Geometry: see drawing. Coordinates: mm, zero at the bounding-box minimum. Give positions to 0.01 mm unless a question says otherwise; leave off trailing zeros. Order: outer loops, then holes, each group sorted by start corner. A loop starts at its lowest first (then second) coordinate and runs counter-clockwise, first axis right, second up. Notation, with made-up numbers: (79, 29.25) - (131, 29.25) arc R25 cw to (131, 47.25) - close; hole circle Ø10 at (57, 36). An arc over 180 degrees is marked (long way). One line per item, written item: value.
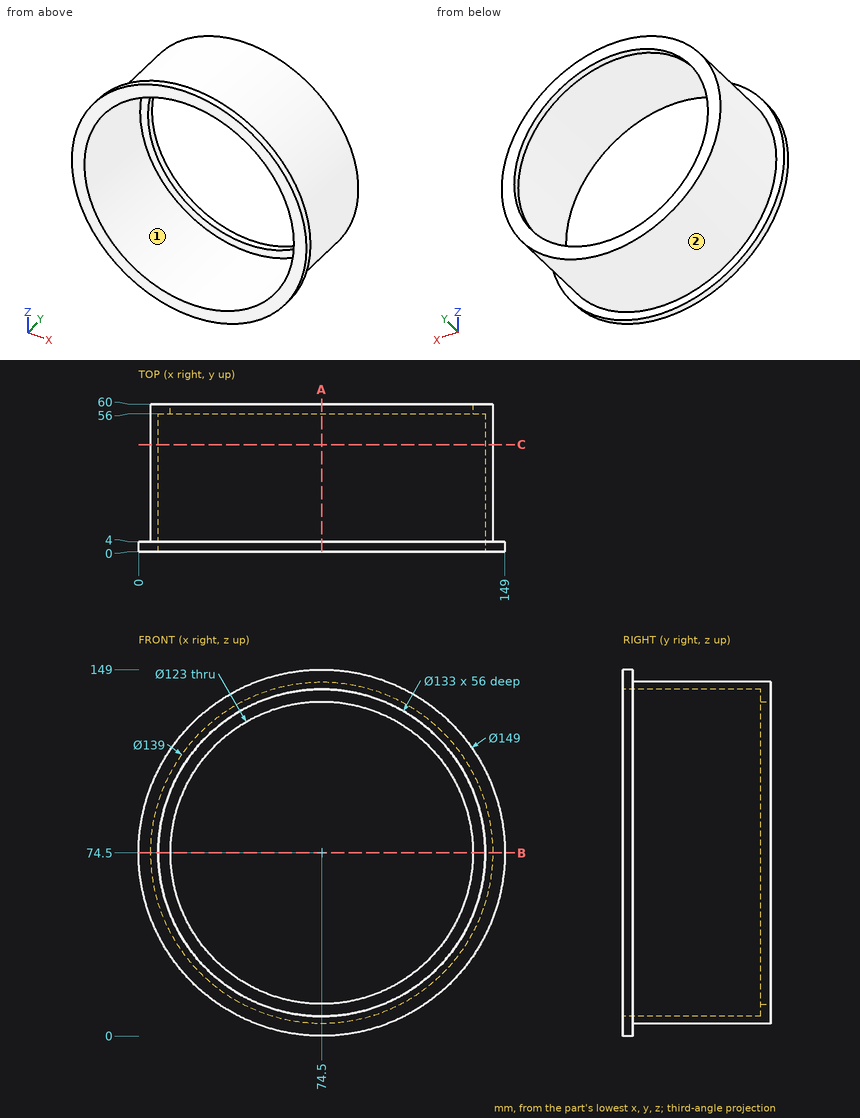
1) Section B-B, the plane z = 74.5. Return loops of the section in (x, y), then the cut area to 3 significant figures.
Answers below:
outline: (0, 0) - (8, 0) - (8, 56) - (13, 56) - (13, 60) - (5, 60) - (5, 4) - (0, 4) - close; (136, 56) - (141, 56) - (141, 0) - (149, 0) - (149, 4) - (144, 4) - (144, 60) - (136, 60) - close
area: 440 mm^2
2) First-contact query: pin 1 (1.5 mm diameter, centred on y = 16, z = 106.5, fed in from -X); pin 2 (1.5 mm diameter, centred on x = 100, y = 38.5, fed in from +Z); pin 3 (5 mm diameter, centred on y = 14, z = 48.5, fed in from -X). Flat tips, straight axial feed; report the tip coordinate or a pass-through.
Answers below:
pin 1: x = 12.42
pin 2: z = 139.44
pin 3: x = 9.09
3) Section A-A, the plane x = 74.5. Return loops of the section in (y, z), then the cut area to 3 significant figures.
Answers below:
outline: (0, 0) - (4, 0) - (4, 5) - (60, 5) - (60, 13) - (56, 13) - (56, 8) - (0, 8) - close; (0, 141) - (56, 141) - (56, 136) - (60, 136) - (60, 144) - (4, 144) - (4, 149) - (0, 149) - close
area: 440 mm^2
4) Material intervals for line 1 along Z through (x, y) = (74.5, 58.4); line 2 along Z through (x, y) = (74.5, 35.5), sorted ascending.
Answers below:
line 1: 5 to 13, 136 to 144
line 2: 5 to 8, 141 to 144
5) Section C-C, the plane y = 43.5. Return loops of the section in (x, z).
Answers below:
outline: circle Ø139 at (74.5, 74.5); hole circle Ø133 at (74.5, 74.5)
6) Mould query, pull axis Z, two halves, no side actions, for the marked faces 1 and 2. Classes: released by +Z, released by -Z, zero draft, split by the parting line, or undercut.
Answers below:
face 1: undercut
face 2: split by the parting line
